from build123d import *

# Parameters (mm, degrees)
SKETCH2_W                = 170
SKETCH2_H                = 153
BOSS_EXTRUDE2_DEPTH      = 5
BOSS_EXTRUDE3_DEPTH      = 85
BOSS_EXTRUDE3_DEPTH_BACK = 85
SKETCH5_W                = 95
SKETCH5_H                = 10.507653329
SKETCH6_W                = 160
SKETCH6_H                = 90
CUT_EXTRUDE1_DEPTH       = 194.724208244
CUT_EXTRUDE3_DEPTH       = 212.54727604
CUT_EXTRUDE3_DEPTH_BACK  = 6
SKETCH7_W                = 30
SKETCH7_H                = 6
CUT_EXTRUDE4_DEPTH       = 10
CUT_EXTRUDE4_DEPTH_BACK  = 6
SKETCH12_W               = 30
SKETCH12_H               = 6
SKETCH26_W               = 19.5
SKETCH26_H               = 5.419548412
BOSS_EXTRUDE5_DEPTH      = 142.492347
SKETCH27_R               = 2.968954814
SKETCH27_R_2             = 3.008499796
SKETCH27_R_3             = 2.994560416
SKETCH27_R_4             = 2.980489199
CUT_EXTRUDE5_DEPTH       = 10
SKETCH31_W               = 89.634159614
SKETCH31_H               = 3
BOSS_EXTRUDE7_DEPTH      = 25
SKETCH32_R               = 3.023319041
SKETCH32_R_2             = 2.995093442
CUT_EXTRUDE7_DEPTH       = 25
SKETCH34_W               = 90
SKETCH34_H               = 3
BOSS_EXTRUDE8_DEPTH      = 25
SKETCH35_R               = 3.039881536
SKETCH35_R_2             = 2.976011356
CUT_EXTRUDE8_DEPTH       = 213.955394622


with BuildPart() as part:
    # Sketch2 → Boss-Extrude2 (new body)
    with BuildSketch(Plane.XY):
        Rectangle(SKETCH2_W, SKETCH2_H)
    extrude(amount=BOSS_EXTRUDE2_DEPTH)

    # Sketch5 → Boss-Extrude3 (add, two sides: drawn at the far end of the back side and taken through both)
    with BuildSketch(Plane(origin=(0, 0, 0), x_dir=(0, 0, -1), z_dir=(1, 0, 0)).offset(-BOSS_EXTRUDE3_DEPTH_BACK)):
        with Locations((-52.5, -71.246173336)):
            Rectangle(SKETCH5_W, SKETCH5_H)
    extrude(amount=BOSS_EXTRUDE3_DEPTH + BOSS_EXTRUDE3_DEPTH_BACK)

    # Sketch6 → Cut-Extrude1 (cut, through all)
    with BuildSketch(Plane(origin=(0, -65.992346671, 0), x_dir=(1, 0, 0), z_dir=(0, 1, 0))):
        with Locations((0.445660274, -49.580451588)):
            Rectangle(SKETCH6_W, SKETCH6_H)
    extrude(amount=-CUT_EXTRUDE1_DEPTH, mode=Mode.SUBTRACT)

    # Sketch7 → Cut-Extrude3 (cut, two sides: drawn at the far end of the back side and taken through both)
    with BuildSketch(Plane(origin=(85, 0, 0), x_dir=(0, 0, -1), z_dir=(1, 0, 0)).offset(-CUT_EXTRUDE3_DEPTH_BACK)):
        with Locations((-65, -68.992346671)):
            Rectangle(SKETCH7_W, SKETCH7_H)
    extrude(amount=CUT_EXTRUDE3_DEPTH + CUT_EXTRUDE3_DEPTH_BACK, mode=Mode.SUBTRACT)

    # Sketch12 → Cut-Extrude4 (cut, two sides: drawn at the far end of the back side and taken through both)
    with BuildSketch(Plane.ZY.offset(85).offset(-CUT_EXTRUDE4_DEPTH_BACK)):
        with Locations((52, -68.992346671)):
            Rectangle(SKETCH12_W, SKETCH12_H)
    extrude(amount=CUT_EXTRUDE4_DEPTH + CUT_EXTRUDE4_DEPTH_BACK, mode=Mode.SUBTRACT)

    # Sketch26 → Boss-Extrude5 (add, through all)
    with BuildSketch(Plane(origin=(0, -65.992346671, 0), x_dir=(1, 0, 0), z_dir=(0, 1, 0))):
        with Locations((-55.25, -97.290225794)):
            Rectangle(SKETCH26_W, SKETCH26_H)
        with Locations((55.25, -97.290225794)):
            Rectangle(SKETCH26_W, SKETCH26_H)
    extrude(amount=BOSS_EXTRUDE5_DEPTH)

    # Sketch27 → Cut-Extrude5 (cut)
    with BuildSketch(Plane.XY.offset(100)):
        with Locations((-55, -43.5)):
            Circle(SKETCH27_R)
        with Locations((-55, 61.5)):
            Circle(SKETCH27_R_2)
        with Locations((55, 61.5)):
            Circle(SKETCH27_R_3)
        with Locations((55, -43.5)):
            Circle(SKETCH27_R_4)
    extrude(amount=-CUT_EXTRUDE5_DEPTH, mode=Mode.SUBTRACT)

    # Sketch31 → Boss-Extrude7 (add)
    with BuildSketch(Plane.XY.offset(100)):
        with Locations((0, -75)):
            Rectangle(SKETCH31_W, SKETCH31_H)
    extrude(amount=BOSS_EXTRUDE7_DEPTH)

    # Sketch32 → Cut-Extrude7 (cut)
    with BuildSketch(Plane(origin=(0, -73.5, 0), x_dir=(1, 0, 0), z_dir=(0, 1, 0))):
        with Locations(Location((-19.817079807, -115, 0), (0, 0, 270))):
            Circle(SKETCH32_R)
        with Locations(Location((19.817079807, -115, 0), (0, 0, 270))):
            Circle(SKETCH32_R_2)
    extrude(amount=-CUT_EXTRUDE7_DEPTH, mode=Mode.SUBTRACT)

    # Sketch34 → Boss-Extrude8 (add)
    with BuildSketch(Plane(origin=(0, 0, 0), x_dir=(-1, 0, 0), z_dir=(0, 0, -1))):
        with Locations((0, -75)):
            Rectangle(SKETCH34_W, SKETCH34_H)
    extrude(amount=BOSS_EXTRUDE8_DEPTH)

    # Sketch35 → Cut-Extrude8 (cut, through all)
    with BuildSketch(Plane(origin=(0, -73.5, 0), x_dir=(1, 0, 0), z_dir=(0, 1, 0))):
        with Locations(Location((-20, 15, 0), (0, 0, 270))):
            Circle(SKETCH35_R)
        with Locations(Location((22.592886771, 15, 0), (0, 0, 270))):
            Circle(SKETCH35_R_2)
    extrude(amount=-CUT_EXTRUDE8_DEPTH, mode=Mode.SUBTRACT)


solid = part.part
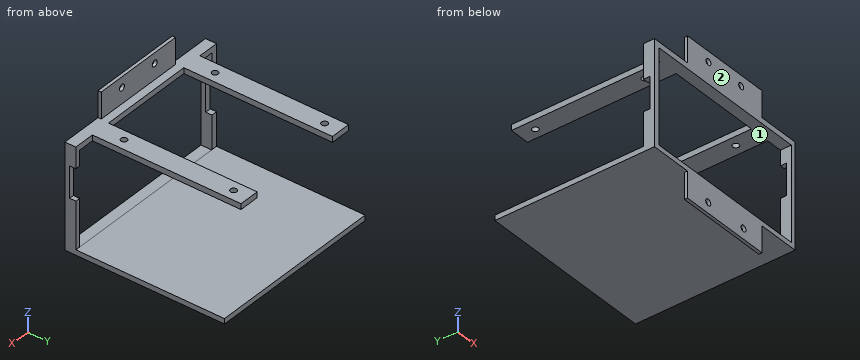
Geometry: final body of the model. Coordinates: model frame, mm. Face numbers are marked on the shaded views. Give positions to 0.01 mm unless a question says otherwise; leave off trailing zeros. Loops run counter-clockwise (first coordinate to the right, second up) from the corner with the lowest first, then second, coordinate; pieces in that order, holes last. Notation, with made-up numbers: (9, 28.5) - (50, 28.5) arc R23 cw to (50, 41.5) - close; hole circle Ø11 at (67, -4). An arc over 180 degrees is marked (long way). Answer as CSV lines item,"result". Start each with the question number.
1. Pin query (flat end, axial travel): P1, Ø2.5, axis at x = -83, z = 28.5, coming from the +Y side; P2, Ø1.5, axis at y = -75.5, z = 118.5, coming from the +X side; P3, Ø1.6, axis at y = 17.5, z = 98.5, coming from the +X side. Return the tip coordinate at first contact, or that it passes through.
2. Section D-D, the plane z = 61.5. Return loops of the section in (x, y).
3. Section B-B, the plane y = 61.5. Return loops of the section in (x, z), plus the area to 3 significant figures.
4. Draft query along Z for the marked faces 1 and 2. Return one class per face: released by +Z, released by -Z, zero draft, split by the parting line, or undercut.
5. Section C-C, the plane x = 55. Return loops of the section in (y, z), plus the area to 3 significant figures.
6. Section A-A, the plane z = 115. Return loops of the section in (x, y).
7. Ray query, L1, parallel to Y at x = 55, z = 97; L2, parallel to X at y = -75.4, z = -15; L3, parallel to X at y = 43, z = 95. Return the intervals inside material, ascending.
Answers:
1,P1,"stops at y = -65.99"
1,P2,"stops at x = 44.82"
1,P3,"stops at x = 65"
2,outline,"(-85, -76.5) - (-79.55, -76.5) - (-79.55, -71.99) - (-85, -71.99) - close; (80.45, -76.5) - (85, -76.5) - (85, -71.99) - (80.45, -71.99) - close"
3,outline,"(-85, 0) - (85, 0) - (85, 5) - (-85, 5) - close; (-65, 94.58) - (-58.01, 94.58) - (-58.01, 100) - (-65, 100) - close; (-51.99, 94.58) - (-45.5, 94.58) - (-45.5, 100) - (-51.99, 100) - close; (45.5, 94.58) - (52.01, 94.58) - (52.01, 100) - (45.5, 100) - close; (57.99, 94.58) - (65, 94.58) - (65, 100) - (57.99, 100) - close"
3,area,"996 mm2"
4,face 1,"undercut"
4,face 2,"zero draft"
5,outline,"(-76.5, 0) - (76.5, 0) - (76.5, 5) - (-65.99, 5) - (-65.99, 4.58) - (-76.5, 4.58) - close; (-76.5, 94.58) - (-46.48, 94.58) - (-46.48, 100) - (-76.5, 100) - close; (-40.52, 94.58) - (58.51, 94.58) - (58.51, 100) - (-40.52, 100) - close; (64.49, 94.58) - (76.5, 94.58) - (76.5, 100) - (64.49, 100) - close"
5,area,"1,530 mm2"
6,outline,"(-44.82, -76.5) - (-22.84, -76.5) - (-22.84, -73.5) - (-44.82, -73.5) - close; (-16.79, -76.5) - (16.82, -76.5) - (16.82, -73.5) - (-16.79, -73.5) - close; (22.81, -76.5) - (44.82, -76.5) - (44.82, -73.5) - (22.81, -73.5) - close"
7,L1,"y = -76.5 to -46.48, -40.52 to 58.51, 64.49 to 76.5"
7,L2,"x = -45 to -23.04, -16.96 to 19.62, 25.57 to 45"
7,L3,"x = -65 to -45.5, 45.5 to 65"
